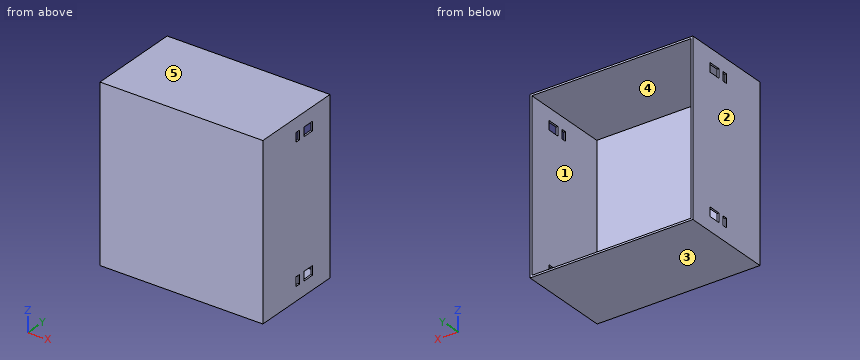
```python
from build123d import *

# Parameters (mm, degrees)
SKETCH_1_W          = 272
SKETCH_1_H          = 286
SKETCH_1_W_2        = 266
SKETCH_1_H_2        = 280
EXTRUDE_1_DEPTH     = 150
SKETCH_2_W          = 272
SKETCH_2_H          = 286
EXTRUDE_2_DEPTH     = 5
SKETCH_3_W          = 15
SKETCH_3_H          = 8
SKETCH_3_H_2        = 20
CUT_EXTRUDE_1_DEPTH = 342.954675359


with BuildPart() as part:
    # 草圖1 → 填料-伸長1 (new body)
    with BuildSketch(Plane(origin=(0, 0, 0), x_dir=(1, 0, 0), z_dir=(0, 1, 0))):
        Rectangle(SKETCH_1_W, SKETCH_1_H)
        Rectangle(SKETCH_1_W_2, SKETCH_1_H_2, mode=Mode.SUBTRACT)
    extrude(amount=EXTRUDE_1_DEPTH)

    # 草圖2 → 填料-伸長2 (add)
    with BuildSketch(Plane.XZ):
        Rectangle(SKETCH_2_W, SKETCH_2_H)
    extrude(amount=EXTRUDE_2_DEPTH)

    # 草圖3 → 除料-伸長1 (cut, through all)
    with BuildSketch(Plane.ZY.offset(136)):
        with Locations((-112.5, 76)):
            Rectangle(SKETCH_3_W, SKETCH_3_H)
        with Locations((-112.5, 100)):
            Rectangle(SKETCH_3_W, SKETCH_3_H_2)
    cut_extrude_1 = extrude(amount=-CUT_EXTRUDE_1_DEPTH, mode=Mode.SUBTRACT)

    # 鏡射1: 除料-伸長1 across plane
    add(cut_extrude_1.mirror(Plane.XY), mode=Mode.SUBTRACT)


solid = part.part
```
The model under review builds one solid part; all positions refer to its coordinate system, in mm. Face numbers are marked on the shaded views. A direction names the side the tool comes from. Round coordinates to 2 decimals unless told otherwise and drop trailing zeros. Write each loop counter-clockwise with the first axis right and the second up, starting at its lowest first coordinate (ties: lowest second). Pieces come first, ordered by that corner, then holes.
(1) We need section B-B on x = -61. Give the boundary of the cut face in (y, z).
(2) Machinability: for the marked faces 4 and 5, which of the approach directions +Z, -Z, +X, -X, +Y, -Y give a long, thin tool a straight path to every point of the face, cutting with its end or side? Answer none if there is none.
(3) We need section A-A on y = 96. Give the boundary of the cut face in (x, z).
(4) Mouldability with a two-part tool opening along X and no side actions: class the marked faces 1, 2 and 3 as +X half, -X half, draft (parallel to the pull), parting line (faces both ways), or undercut.
(5) We need section C-C on y = 131.5. Give the boundary of the cut face in (x, z).
(6) Wall thickness on L1, parallel to Z at x = -7.5, y = 46; L2, parallel to X at y = 120.5, z = 67.5; L3, parallel to Y at x = 105, z = -35: over which ranges is each line inside the solid? List them lowest first.
(7) We need section D-D on z = -88. Give the boundary of the cut face in (x, y).
Findings below:
1. outline: (-5, -143) - (150, -143) - (150, -140) - (0, -140) - (0, 140) - (150, 140) - (150, 143) - (-5, 143) - close
2. face 4: +Y
2. face 5: +Z, +X, -X, +Y, -Y
3. outline: (-136, -143) - (136, -143) - (136, -120) - (133, -120) - (133, -140) - (-133, -140) - (-133, -120) - (-136, -120) - close; (-136, -105) - (-133, -105) - (-133, 105) - (-136, 105) - close; (-136, 120) - (-133, 120) - (-133, 140) - (133, 140) - (133, 120) - (136, 120) - (136, 143) - (-136, 143) - close; (133, -105) - (136, -105) - (136, 105) - (133, 105) - close
4. face 1: undercut
4. face 2: -X half
4. face 3: draft
5. outline: (-136, -143) - (136, -143) - (136, 143) - (-136, 143) - close; hole (-133, -140) - (133, -140) - (133, 140) - (-133, 140) - close
6. L1: z = -143 to -140, 140 to 143
6. L2: x = -136 to -133, 133 to 136
6. L3: y = -5 to 0
7. outline: (-136, -5) - (136, -5) - (136, 150) - (133, 150) - (133, 0) - (-133, 0) - (-133, 150) - (-136, 150) - close
